The listing builds one solid part. Answer for the finished solid, in the listing's coordinates (mm). A direction names the side the tool comes from. Give positions to 0.01 mm unless a question says otherwise; leave off trailing zeros. Loops run counter-clockwise (first coordinate to the right, second up) from the corner with the lowest first, then second, coordinate; pieces in that order, holes last. Notation, with made-up numbers: (32.25, 42) - (83.25, 42) arc R11 cw to (83.25, 57) - close; hole circle Ø6 at (-3.5, 67). An arc over 180 degrees is marked (long way). Write item = value, one per line. Start each with the question number.
1) The part is cut by section C-C on x = 1.5. State how many separate pieces and enclosed holes the cut face has, plus the area to 3 significant figures.
2) The part is cut by section D-D on y = 0. Write down the section's boundary in (x, z), plus the area to 3 significant figures.
3) The mould has two halves that part along Z. Classify faces 4 (the cylindrical face through (2, 11, 0)), 5 (the flat face through (0, 10, 3.7)), 6 (the flat face through (0, 18, -1)): +Z half, -Z half, draft (parallel to the pull), parting line (faces both ways), or undercut.
4) The part is cut by section A-A on z = 4.75. Write down the section's boundary in (x, y), plus the area to 3 significant figures.
5) Which of the six approach directions +Z, -Z, +X, -X, +Y, -Y give full straight-line access (tool end or side, diameter ignored) to faces 1 (the cylindrical face through (1.96, 35.57, -0.28)), 2 (the flat face through (-4, 12, 2)), 3 (the flat face through (-6, -13.5, 2))?
6) The part is cut by section B-B on y = -12.2. Write down the section's boundary in (x, z).
7) Flat-ended cylindrical pins translate along their axes: P1, Ø5, axis at x = -4, y = 19.5, coming from the +Z side; P2, Ø3.5, axis at y = 12.5, z = 0, coming from the -X side; P3, Ø5, axis at x = 1.5, y = -12.2, coming from the -Z side. Find the tip coordinate at first contact, or state that the pin passes through.
8) Consider probe 1 along Y at (x, z) = (-8, 0.5); probe 2 along X at (y, z) = (0, 2.25); probe 3 along Z at (x, y) = (4.75, 12.5). Determine where each line is inside the solid, lowest interval first.
from build123d import *

# Parameters (mm, degrees)
EXTRUSION1_DEPTH                                = 8
EXTRUSION1_DEPTH_BACK                           = 9
ESQUISSE1_W                                     = 10
ESQUISSE1_H                                     = 57
ESQUISSE1_R                                     = 1.5
ESQUISSE2_R                                     = 6
ESQUISSE2_W                                     = 5
ESQUISSE2_H                                     = 8
ESQUISSE2_H_2                                   = 7.5
ENL_V_MAT_EXTRU_1_DEPTH                         = 39.431757701
ESQUISSE3_W                                     = 3.8
ESQUISSE3_H                                     = 39.8
ESQUISSE3_W_2                                   = 2.5
ESQUISSE3_H_2                                   = 10
ENL_V_MAT_EXTRU_2_DEPTH                         = 41.512343798
CHAMBRAGE_POUR_VIS_T_TE_CYLINDRIQUE_D           = 4.2
CHAMBRAGE_POUR_VIS_T_TE_CYLINDRIQUE_CBORE_D     = 7
CHAMBRAGE_POUR_VIS_T_TE_CYLINDRIQUE_CBORE_DEPTH = 4.5


with BuildPart() as part:
    # Esquisse1 → Extrusion1 (new, two sides: drawn at the far end of the back side and taken through both)
    with BuildSketch(Plane(origin=(0, 0, 0), x_dir=(0, 0, -1), z_dir=(1, 0, 0)).offset(-EXTRUSION1_DEPTH_BACK)):
        with Locations((-2.5, 7.5)):
            Rectangle(ESQUISSE1_W, ESQUISSE1_H)
        with Locations((0, 12.5)):
            Circle(ESQUISSE1_R, mode=Mode.SUBTRACT)
        with Locations((0, -17.5)):
            Circle(ESQUISSE1_R, mode=Mode.SUBTRACT)
    extrude(amount=EXTRUSION1_DEPTH + EXTRUSION1_DEPTH_BACK)

    # Esquisse2 → Enlèv. mat.-Extru.1 (cut, through all)
    with BuildSketch(Plane(origin=(0, 0, -2.5), x_dir=(-1, 0, 0), z_dir=(0, 0, -1))):
        with Locations(Location((0, 0, 0), (0, 0, 90))):
            Circle(ESQUISSE2_R)
        with Locations((6.5, 12.5)):
            Rectangle(ESQUISSE2_W, ESQUISSE2_H)
        with Locations((6.5, -17.25)):
            Rectangle(ESQUISSE2_W, ESQUISSE2_H_2)
    extrude(amount=-ENL_V_MAT_EXTRU_1_DEPTH, mode=Mode.SUBTRACT)

    # Esquisse3 → Enlèv. mat.-Extru.2 (cut, through all)
    with BuildSketch(Plane(origin=(8, 0, 0), x_dir=(0, 0, -1), z_dir=(1, 0, 0))):
        with Locations((-5.6, 9.95)):
            Rectangle(ESQUISSE3_W, ESQUISSE3_H)
        with Locations((1.25, 23)):
            Rectangle(ESQUISSE3_W_2, ESQUISSE3_H_2)
    extrude(amount=-ENL_V_MAT_EXTRU_2_DEPTH, mode=Mode.SUBTRACT)

    # Chambrage pour vis à tête cylindrique à 6 pans creux (ou vis CHC) M46 (through all)
    with Locations(Plane(origin=(0, 0, -2.5), x_dir=(-1, 0, 0), z_dir=(0, 0, -1))):
        with Locations((-1.5, -12.2), (-1.5, 32.1)):
            CounterBoreHole(CHAMBRAGE_POUR_VIS_T_TE_CYLINDRIQUE_D / 2, CHAMBRAGE_POUR_VIS_T_TE_CYLINDRIQUE_CBORE_D / 2, CHAMBRAGE_POUR_VIS_T_TE_CYLINDRIQUE_CBORE_DEPTH)


solid = part.part
Answer below:
q1.separate_pieces = 4
q1.enclosed_holes = 2
q1.area = 198 mm2
q2.outline = (-9, -2.5) - (-6, -2.5) - (-6, 3.7) - (-9, 3.7) - close; (6, -2.5) - (8, -2.5) - (8, 3.7) - (6, 3.7) - close
q2.area = 31.0 mm2
q3.face_4 = undercut
q3.face_5 = +Z half
q3.face_6 = draft
q4.outline = (-9, -13.5) - (-4, -13.5) - (-4, -21) - (8, -21) - (8, -9.95) - (-9, -9.95) - close; (-9, 29.85) - (8, 29.85) - (8, 36) - (-9, 36) - close; hole circle Ø4.2 at (1.5, -12.2); hole circle Ø4.2 at (1.5, 32.1)
q4.area = 227 mm2
q5.face_1 = -Z
q5.face_2 = +Z, -Z, -X
q5.face_3 = +Z, -Z, -X, -Y
q6.outline = (-9, -2.5) - (-2, -2.5) - (-2, 2) - (-0.6, 2) - (-0.6, 7.5) - (-9, 7.5) - close; (3.6, 2) - (5, 2) - (5, -2.5) - (8, -2.5) - (8, 7.5) - (3.6, 7.5) - close
q7.P1 = 3.7
q7.P2 = -4
q7.P3 = 2
q8.probe_1 = -13.5 to 8.5, 16.5 to 36
q8.probe_2 = -9 to -6, 6 to 8
q8.probe_3 = -2.5 to -1.5, 1.5 to 3.7
